```python
from build123d import *

# Parameters (mm, degrees)
SKETCH001_W        = 1.5
SKETCH001_H        = 10
POCKET_DEPTH       = 4
POLARPATTERN_COUNT = 5


with BuildPart() as part:
    # Sketch → Revolution (revolve)
    with BuildSketch(Plane.XZ):
        with BuildLine():
            Line((16, 0), (16, 2))
            ThreePointArc((16, 2), (13.071068, 9.071068), (6, 12))
            Line((3.5, 12), (6, 12))
            Line((3.5, 7.7), (3.5, 12))
            Line((1.8, 6), (3.5, 7.7))
            Line((1.8, 6), (1.8, 0))
            Line((1.8, 0), (16, 0))
        make_face()
    revolve(axis=Axis((0, 0, 0), (0, 0, 1)))

    # Sketch001 (on Face2 of Revolution) → Pocket (cut)
    with BuildSketch(Plane(origin=(0, 0, 0), x_dir=(1, 0, 0), z_dir=(0, 0, -1))):
        with Locations((0, 8.5)):
            Rectangle(SKETCH001_W, SKETCH001_H)
    pocket = extrude(amount=-POCKET_DEPTH, mode=Mode.SUBTRACT)

    # PolarPattern: Pocket ×5 about axis
    polarpattern_axis = Axis((0, 0, 0), (0, 0, -1))
    for i in range(1, POLARPATTERN_COUNT):
        add(pocket.rotate(polarpattern_axis, i * 360 / POLARPATTERN_COUNT), mode=Mode.SUBTRACT)


solid = part.part
```
Here's how the part is built. I have some questions about the finished solid (model axes, mm). A direction names the side the tool comes from. Give positions to 0.01 mm unless a question says otherwise; leave off trailing zeros. Put each result on its own line as item: value. Start each with the question number.
Item 1: I need wall thicknesses on L1, parallel to Y at x = 0, z = 2.15; L2, parallel to Y at x = -4, z = 1.5; L3, parallel to X at y = 5.5, z = 2.25. Which ranges of each line are inside material? Lowest first, please. Write a range as from..to.
Item 2: Will these pins go through, and if not, where does the flat tip stop? pin 1 (1.5 mm diameter, centred on x = 8.5, z = 8, fed in from -Y); pin 2 (3 mm diameter, centred on y = -6.5, z = 2.5, fed in from -X); pin 3 (4 mm diameter, centred on x = 0, y = 0, fed in from +Z).
Item 3: On a 3-axis mill with a long thin cutter (end or side, diameter ignored), from which of +Z, -Z, +X, -X, +Y, -Y can I reach the whole of each face in a straight line? I mean faces 1 (the cylindrical face through (1.717, 0.541, 2.958)), 2 (the flat face through (0, -3.5, 2)). Say none if no direction works.
Item 4: Thinking about a two-plate mould opening in X: for faces 3 (the conical face through (1.818, 0.573, 6.106)), 4 (the flat face through (-3, -3, 12)), 5 (the cylindrical face through (-3.47, -15.62, 1.01)), which applies, +X half, -X half, draft (parallel to the pull), parting line (faces both ways), or undercut?
Values:
1. L1: -16..-13.5, -3.5..-1.8, 1.8..16
1. L2: -15.49..-2.09, -0.51..4.23, 6.78..15.49
1. L3: -15.02..-4.92, -3.07..3.07, 4.92..15.02
2. pin 1: y = -11.96
2. pin 2: x = -15.19
2. pin 3: z = 6.2
3. face 1: +Z, -Z
3. face 2: -Z
4. face 3: undercut
4. face 4: draft
4. face 5: parting line
